```python
from build123d import *

# Parameters (mm, degrees)
F0_W     = 97
F0_H     = 84
F1_DEPTH = 98
F2_T     = -2
F3_W     = 72
F3_H     = 31
F3_R     = 2.5
F3_R_2   = 3
F4_DEPTH = 2
F5_W     = 10
F5_H     = 10
F5_R     = 2.25
F6_DEPTH = 10
F7_R     = 2
F8_DEPTH = 25.4


with BuildPart() as f1:
    # F0 (on Front) → F1 (new body)
    with BuildSketch(Plane.XZ):
        Rectangle(F0_W, F0_H)
    extrude(amount=F1_DEPTH)

    # F2
    f2_openings = [f1.faces().sort_by_distance(p)[0] for p in [
        (0, 0, 0),
    ]]
    offset(amount=F2_T, openings=f2_openings)

    # F3 (on face) → F4 (cut, through all)
    with BuildSketch(Plane.XZ.offset(98)):
        with BuildLine():
            ThreePointArc((-4.5, -7.75), (-19.5, 0), (-34.5, -7.75))
            Line((-34.5, -7.75), (-34.5, -27.75))
            ThreePointArc((-34.5, -27.75), (-19.5, -35.5), (-4.5, -27.75))
            Line((-4.5, -27.75), (-4.5, -7.75))
        make_face()
        with Locations((0, 22.5)):
            Rectangle(F3_W, F3_H)
        with BuildLine():
            Line((34.5, -27.75), (34.5, -7.75))
            ThreePointArc((34.5, -7.75), (19.5, 0), (4.5, -7.75))
            Line((4.5, -7.75), (4.5, -27.75))
            ThreePointArc((4.5, -27.75), (19.5, -35.5), (34.5, -27.75))
        make_face()
        with Locations((0, -17.75)):
            Circle(F3_R)
        with Locations((-41.8, -17.75)):
            Circle(F3_R_2)
        with Locations((41.8, -17.75)):
            Circle(F3_R_2)
    extrude(amount=-F4_DEPTH, mode=Mode.SUBTRACT)

    # F5 (on face) → F6 (join)
    with BuildSketch(Plane(origin=(0, 0, 0), x_dir=(-1, 0, 0), z_dir=(0, 1, 0))):
        with Locations((-41.5, 35)):
            Rectangle(F5_W, F5_H)
        with Locations((-41.5, 35)):
            Circle(F5_R, mode=Mode.SUBTRACT)
        with Locations((41.5, 35)):
            Rectangle(F5_W, F5_H)
        with Locations((41.5, 35)):
            Circle(F5_R, mode=Mode.SUBTRACT)
        with Locations((-41.5, -35)):
            Rectangle(F5_W, F5_H)
        with Locations((-41.5, -35)):
            Circle(F5_R, mode=Mode.SUBTRACT)
        with Locations((41.5, -35)):
            Rectangle(F5_W, F5_H)
        with Locations((41.5, -35)):
            Circle(F5_R, mode=Mode.SUBTRACT)
    extrude(amount=-F6_DEPTH)

    # F7
    f7_edges = [f1.edges().sort_by_distance(p)[0] for p in [
        (36.5, -5, 40),
        (46.5, -5, 30),
        (-36.5, -5, 40),
        (-46.5, -5, 30),
        (-36.5, -5, -40),
        (-46.5, -5, -30),
        (36.5, -5, -40),
        (46.5, -5, -30),
        (36.5, -5, 30),
        (36.5, -5, -30),
        (-36.5, -5, 30),
        (-36.5, -5, -30),
    ]]
    fillet(f7_edges, radius=F7_R)

    # F8 (add): a face of the model
    f8_faces = [f1.faces().sort_by_distance(p)[0] for p in [
        (-41.5, -10, -30.1697056275),
    ]]
    extrude(f8_faces, amount=F8_DEPTH)


solid = f1.part
```
The listing builds one solid part. Answer for the finished solid, in the listing's coordinates (mm). A direction names the side the tool comes from. Give positions to 0.01 mm unless a question says otherwise; leave off trailing zeros. Order: outer loops, then holes, each group sorted by start corner. A loop starts at its lowest first (then second) coordinate and runs counter-clockwise, first axis right, second up.
1) Find section A-A on z = 35. Write down the section's boundary in (x, y), then the cut area to 3 significant figures.
Reported:
outline: (-48.5, -98) - (-36, -98) - (-36, -96) - (-46.5, -96) - (-46.5, -10) - (-43.75, -10) - (-43.75, 0) - (-48.5, 0) - close; (-39.25, -10) - (-36.5, -10) - (-36.5, 0) - (-39.25, 0) - close; (36, -98) - (48.5, -98) - (48.5, 0) - (43.75, 0) - (43.75, -10) - (46.5, -10) - (46.5, -96) - (36, -96) - close; (36.5, -10) - (39.25, -10) - (39.25, 0) - (36.5, 0) - close
area: 544 mm2
2) Find section C-C on z = -17.75. Write down the section's boundary in (x, y).
Reported:
outline: (-48.5, -98) - (-44.8, -98) - (-44.8, -96) - (-46.5, -96) - (-46.5, 0) - (-48.5, 0) - close; (-38.8, -98) - (-34.5, -98) - (-34.5, -96) - (-38.8, -96) - close; (-4.5, -98) - (-2.5, -98) - (-2.5, -96) - (-4.5, -96) - close; (2.5, -98) - (4.5, -98) - (4.5, -96) - (2.5, -96) - close; (34.5, -98) - (38.8, -98) - (38.8, -96) - (34.5, -96) - close; (44.8, -98) - (48.5, -98) - (48.5, 0) - (46.5, 0) - (46.5, -96) - (44.8, -96) - close
3) For faces 1 (the face through (-19.3, -97, 0)), 2 (the face through (-41.7, -35.4, -32.6)), 3 (the face through (41.79, -4.93, -32.77)), determine the directions among +Z, -Z, +X, -X, +Y, -Y from which every point of the face is accessible in a straight line to the end or side of a thin tool.
Reported:
face 1: +Y, -Y
face 2: none
face 3: +Y
4) Find section B-B on x = 0. Write down the section's boundary in (y, z), then the cut area to 3 significant figures.
Reported:
outline: (-98, -42) - (0, -42) - (0, -40) - (-96, -40) - (-96, -20.25) - (-98, -20.25) - close; (-98, -15.25) - (-96, -15.25) - (-96, 7) - (-98, 7) - close; (-98, 38) - (-96, 38) - (-96, 40) - (0, 40) - (0, 42) - (-98, 42) - close
area: 480 mm2
5) Consider line 1 along Z through (x, y) = (42.5, -89); line 2 along X through (y, z) = (-86.5, -0.5); line 3 along Z through (x, y) = (41.8, -96.35). Determine where each line is inside the solid, lowest interval first.
Reported:
line 1: z = -42 to -40, 40 to 42
line 2: x = -48.5 to -46.5, 46.5 to 48.5
line 3: z = -42 to -20.75, -14.75 to 42
6) Find section D-D on y = -26.5. Write down the section's boundary in (x, z), then the cut area to 3 significant figures.
Reported:
outline: (-48.5, -42) - (48.5, -42) - (48.5, 42) - (-48.5, 42) - close; hole (-46.5, -28) arc R2 ccw to (-44.5, -30) - (-38.5, -30) arc R2 cw to (-36.5, -32) - (-36.5, -38) arc R2 ccw to (-34.5, -40) - (46.5, -40) - (46.5, 40) - (-46.5, 40) - close; hole circle Ø4.5 at (-41.5, -35)
area: 793 mm2
7) Determine the mould class of faces 4 (the face through (19.7, -97, 0)), 5 (the face through (-1, -98, -9)), 6 (the face through (-1, -48, -42)), 7 (the face through (41.79, -4.93, 37.23)) for opening direction Z: pulls with the +Z half, pulls with the -Z half, needs draft (parallel to the pull), parting line crosses it, or undercut.
Reported:
face 4: undercut
face 5: needs draft
face 6: pulls with the -Z half
face 7: undercut
8) Given P1, Ø4, axis at x = 41.5, z = 35, coming from the +Y side, flat-ended and moving along its own axis, determine where the tip first touches the part or whether it passes through.
Reported:
P1: stops at y = -96
